```python
from build123d import *

# Parameters (mm, degrees)
SKETCH1_W           = 20
SKETCH1_H           = 155.5
BOSS_EXTRUDE1_DEPTH = 10
SKETCH2_R           = 9
BOSS_EXTRUDE2_DEPTH = 2.5
SKETCH3_R           = 1.7
CUT_EXTRUDE1_DEPTH  = 80.380806874
FILLET1_R           = 10


with BuildPart() as part:
    # Sketch1 → Boss-Extrude1 (new body)
    with BuildSketch(Plane.XY):
        Rectangle(SKETCH1_W, SKETCH1_H)
    extrude(amount=BOSS_EXTRUDE1_DEPTH)

    # Sketch2 → Boss-Extrude2 (add)
    with BuildSketch(Plane(origin=(0, 0, 0), x_dir=(-1, 0, 0), z_dir=(0, 0, -1))):
        with Locations(Location((0, 65, 0), (0, 0, 180))):
            Circle(SKETCH2_R)
        with Locations(Location((0, -65, 0), (0, 0, 180))):
            Circle(SKETCH2_R)
    extrude(amount=BOSS_EXTRUDE2_DEPTH)

    # Sketch3 → Cut-Extrude1 (cut, through all)
    with BuildSketch(Plane(origin=(0, 0, -2.5), x_dir=(-1, 0, 0), z_dir=(0, 0, -1))):
        with Locations((0, 65)):
            Circle(SKETCH3_R)
        with Locations((0, -65)):
            Circle(SKETCH3_R)
    extrude(amount=-CUT_EXTRUDE1_DEPTH, mode=Mode.SUBTRACT)

    # Fillet1
    fillet1_edges = [part.edges().sort_by_distance(p)[0] for p in [
        (10, -77.75, 5),
        (-10, -77.75, 5),
        (-10, 77.75, 5),
        (10, 77.75, 5),
    ]]
    fillet(fillet1_edges, radius=FILLET1_R - 0.0001)  # a hair under: the kernel refuses the full size


solid = part.part
```
The listing builds one solid part. Answer for the finished solid, in the listing's coordinates (mm). A direction names the side the tool comes from. Coordinates: 2 decimals unless noted, no trailing zeros. Write each loop counter-clockwise with the first axis right and the second up, starting at its lowest first coordinate (ties: lowest second). Pieces come first, ordered by that corner, then holes. Notation, with made-up numbers: (-8.5, 69) - (5.5, 69) arc R10 cw to (5.5, 75) - close; hole circle Ø7 at (59, 30.5). An arc over 180 degrees is marked (long way). Return JSON: item names as keys, results as strings. Group by question number.
Q1. Flat-ended cylindrical pins translate along their axes: pin 1 Ø10 at (x, y) = (3, 30.5) entering from -Z; pin 2 Ø4 at (x, y) = (0, 65) entering from +Z; pin 3 Ø2 at (x, z) = (8, 4.5) entering from +Y; pin 4 Ø5 at (x, z) = (-7.5, 7.5) entering from +Y. Find the tip coordinate at first contact, or state that the pin passes through.
Q2. Find the intervals of material crossed by line 1 along Y through (x, z) = (0, 3.5); line 2 along X through (y, z) = (65, 3.5); line 3 along Z through (x, y) = (7, -58), in increasing order. Write a range as [from, to].
Q3. The part is cut by section A-A on z = 4.25. State how many separate pieces and enclosed holes the cut face has, and give its area (3 significant figures).
Q4. Which of the six approach directions +Z, -Z, +X, -X, +Y, -Y give full straight-line access (tool end or side, diameter ignored) to faces 1 (the cylindrical face through (-1.951, -56.214, -1.232)), 2 (the flat face through (2, -65, -2.5))?
Q5. The part is cut by section C-C on x = 3.5. Write down the section's boundary in (y, z).
Q6. For a pull along X with two mould halves and no side action, classify faces 3 (the cylindrical face through (6.99, 74.9, 5.07)), 4 (the cylindrical face through (0.221, -63.314, 3.662)), 5 (the flat face through (0, 1, 0)) as +X half, -X half, draft (parallel to the pull), parting line (faces both ways), or undercut.
Q7. The part is cut by section D-D on y = 0.5. Write down the section's boundary in (x, z).
Q8. The part is cut by section B-B on y = -65. Write down the section's boundary in (x, z), and give its area (4 significant figures).
Evaluation:
{
 "1": {"pin 1": "stops at z = 0", "pin 2": "stops at z = 10", "pin 3": "stops at y = 74.89", "pin 4": "stops at y = 76.41"},
 "2": {"line 1": "y = [-77.75, -66.7], [-63.3, 63.3], [66.7, 77.75]", "line 2": "x = [-10, -1.7], [1.7, 10]", "line 3": "z = [0, 10]"},
 "3": {"separate pieces": "1", "enclosed holes": "2", "area": "3,010 mm2"},
 "4": {"face 1": "-Z", "face 2": "-Z, +X, -X, +Y, -Y"},
 "5": {"outline": "(-77.12, 0) - (-73.29, 0) - (-73.29, -2.5) - (-56.71, -2.5) - (-56.71, 0) - (56.71, 0) - (56.71, -2.5) - (73.29, -2.5) - (73.29, 0) - (77.12, 0) - (77.12, 10) - (-77.12, 10) - close"},
 "6": {"face 3": "+X half", "face 4": "undercut", "face 5": "draft"},
 "7": {"outline": "(-10, 0) - (10, 0) - (10, 10) - (-10, 10) - close"},
 "8": {"outline": "(-10, 0) - (-9, 0) - (-9, -2.5) - (-1.7, -2.5) - (-1.7, 10) - (-10, 10) - close; (1.7, -2.5) - (9, -2.5) - (9, 0) - (10, 0) - (10, 10) - (1.7, 10) - close", "area": "202.5 mm2"}
}
